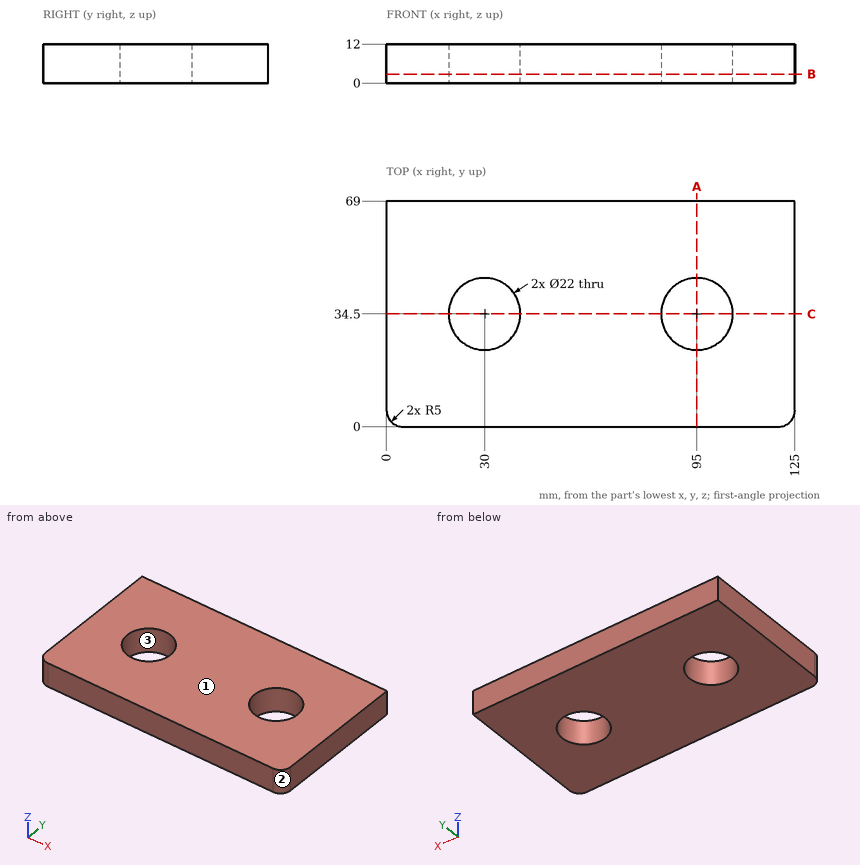
Design review of the part shown in the three views and the two pictorial views. Dimensions are in mm from the part's minimum x, y and z. Round coordinates to 2 decimals unless told otherwise and drop trailing zeros. Loops run counter-clockwise (first coordinate to the right, second up) from the corner with the lowest first, then second, coordinate; pieces in that order, holes last.
1) Consider section B-B on z = 2.75. State the section outline as (x, y) points, then the cut area to 3 significant figures.
Values follow:
outline: (0, 5) arc R5 ccw to (5, 0) - (120, 0) arc R5 ccw to (125, 5) - (125, 69) - (0, 69) - close; hole circle Ø22 at (30, 34.5); hole circle Ø22 at (95, 34.5)
area: 7,850 mm2
2) The part is to be moulded in two halves that separate along X. For the marked faces 1, 2 and 3, say which applies: pulls with the +X half, pulls with the -X half, needs draft (parallel to the pull), parting line crosses it, or undercut.
Values follow:
face 1: needs draft
face 2: pulls with the +X half
face 3: undercut
3) Consider section C-C on y = 34.5. State the section outline as (x, z) points.
Values follow:
outline: (0, 0) - (19, 0) - (19, 12) - (0, 12) - close; (41, 0) - (84, 0) - (84, 12) - (41, 12) - close; (106, 0) - (125, 0) - (125, 12) - (106, 12) - close
4) Consider section A-A on x = 95. State the section outline as (y, z) points, then the cut area to 3 significant figures.
Values follow:
outline: (0, 0) - (23.5, 0) - (23.5, 12) - (0, 12) - close; (45.5, 0) - (69, 0) - (69, 12) - (45.5, 12) - close
area: 564 mm2
5) Wall thickness on line 1 along Y through (x, z) = (30, 4.5); line 2 along X through (y, z) = (44.5, 1.25); line 3 along X through (y, z) = (37.5, 8): over which ranges is each line inside the solid? List them lowest first.
Values follow:
line 1: y = 0 to 23.5, 45.5 to 69
line 2: x = 0 to 25.42, 34.58 to 90.42, 99.58 to 125
line 3: x = 0 to 19.42, 40.58 to 84.42, 105.58 to 125
